from build123d import *

# Parameters (mm, degrees)
F1_DEPTH = 7.5
F3_D     = 6.6
F3_DEPTH = 4
F3_TIP   = 1.9828400428


# Not quite as in the source:
# - a pattern or mirror of a feature is missing from the dataset's text; its kind, count and spacing are read off the source's solid


with BuildPart() as f1:
    # F0 (on Right) → F1 (new body, symmetric)
    with BuildSketch(Plane.YZ):
        with BuildLine():
            Line((19.0101097905, 11), (-19.0101097905, 11))
            ThreePointArc((-19.0101097905, 11), (-30.0101097905, 0), (-19.0101097905, -11))
            Line((-19.0101097905, -11), (19.0101097905, -11))
            ThreePointArc((19.0101097905, -11), (30.0101097905, 0), (19.0101097905, 11))
        make_face()
        with BuildLine():
            Line((16.508441914, -7.5), (-16.508441914, -7.5))
            ThreePointArc((-16.508441914, -7.5), (0, -2.3140263028), (16.508441914, -7.5))
        make_face(mode=Mode.SUBTRACT)
        with BuildLine():
            ThreePointArc((-19.0101097905, -7.5), (-26.5101097905, 0), (-19.0101097905, 7.5))
            ThreePointArc((-19.0101097905, 7.5), (0, 0.8140263028), (19.0101097905, 7.5))
            ThreePointArc((19.0101097905, 7.5), (26.5101097905, 0), (19.0101097905, -7.5))
            ThreePointArc((19.0101097905, -7.5), (0, -0.8140263028), (-19.0101097905, -7.5))
        make_face(mode=Mode.SUBTRACT)
        with BuildLine():
            ThreePointArc((16.508441914, 7.5), (0, 2.3140263028), (-16.508441914, 7.5))
            Line((-16.508441914, 7.5), (16.508441914, 7.5))
        make_face(mode=Mode.SUBTRACT)
    extrude(amount=F1_DEPTH, both=True)

    # F3
    with Locations(Plane.XY.offset(11)):
        with Locations((0, 0)):
            f3 = Hole(F3_D / 2, depth=F3_DEPTH)
            with Locations((0, 0, -(F3_DEPTH + F3_TIP / 2))):  # 118° drill point
                Cone(0, F3_D / 2, F3_TIP, mode=Mode.SUBTRACT)

    # F3_copies: F3 across plane
    add(f3.mirror(Plane(origin=(0, 0, 0), x_dir=(-1, 0, 0), z_dir=(0, 0, -1))), mode=Mode.SUBTRACT)


solid = f1.part
For this review, take the finished solid that the model builds, in its own axes (mm). A direction names the side the tool comes from. Round coordinates to 2 decimals unless told otherwise and drop trailing zeros. Order: outer loops, then holes, each group sorted by start corner. A loop starts at its lowest first (then second) coordinate and runs counter-clockwise, first axis right, second up. Notation, with made-up numbers: M -27,-1.5 L -7,-1.5 A24 cw -7,35.5 Z; hole C 29.25,-20.5 d5. An arc over 180 degrees is marked long. Use a Markdown table: item, result. Add a question column.
Item 1: Mouldability with a two-part tool opening along Z and no side actions: class faces 6 (the cylindrical face through (0.105, 0.288, -0.815)), 7 (the cylindrical face through (0.105, -30.007, 0.242)), 8 (the flat face through (-7.5, 0, -2)) as released by +Z, released by -Z, zero draft, split by the parting line, or undercut.
Item 2: To check wall thickness, follow line 1 along Z through (x, y) = (4.75, -0.5); line 2 along Y through (x, z) = (-4.75, -6.75); line 3 along Y through (x, z) = (1.75, 0). State the ranges of each line that lie inside material, in increasing order.
Item 3: Add section C-C, the plane x = 0. Give the boundary of the cut face in (y, z), then the cut area to 3 significant figures.
Item 4: Add section A-A, the plane z = 0. Give the boundary of the cut face in (x, y), then the cut area to 3 significant figures.
Item 5: Insertion check: pin 1 (1 mm diameter, centred on x = 4.5, z = 8.5, fed in from +Y); pin 2 (4 mm diameter, centred on x = 5, z = -3, fed in from +Y); pin 3 (4 mm diameter, centred on x = 0, y = 0, fed in from -Z). Each pin has a flat end and moves straight along its axis. Give the tip position at first contact, or say it passes through.
Item 6: Add section B-B, the plane y = 0. Give the boundary of the cut face in (x, z).
Item 7: Tool access review of faces 1 (the cylindrical face through (2.43, 2.23, 9.23)), 2 (the flat face through (3.44, -0.27, -11)), 3 (the cylindrical face through (0.11, 26.51, 0.16)), 4 (the flat face through (7.5, 0, -2)), 5 (the cylindrical face through (2.43, 2.23, -9.23)): name each direction out of +Z, -Z, +X, -X, +Y, -Y from which nothing blocks a thin tool from reaching the whole face with its end or side.
Item 8: Add section D-D, the plane z = -6.5. Give the boundary of the cut face in (x, y), then the cut area to 3 significant figures.
Geometry results:
| question | item | result |
|---|---|---|
| 1 | face 6 | undercut |
| 1 | face 7 | split by the parting line |
| 1 | face 8 | zero draft |
| 2 | line 1 | z = -11 to -7.5, -2.32 to -0.82, 0.82 to 2.32, 7.5 to 11 |
| 2 | line 2 | y = -27.7 to -22.28, -18.04 to -15.38, 15.38 to 18.04, 22.28 to 27.7 |
| 2 | line 3 | y = -30.01 to -26.51, 26.51 to 30.01 |
| 3 | outline | M -19.01,-11 L -3.3,-11 L -3.3,-7.5 L -16.51,-7.5 A28.87 cw 16.51,-7.5 L 3.3,-7.5 L 3.3,-11 L 19.01,-11 A11 ccw 19.01,11 L 3.3,11 L 3.3,7.5 L 16.51,7.5 A28.87 cw -16.51,7.5 L -3.3,7.5 L -3.3,11 L -19.01,11 A11 ccw Z; hole M -19.01,-7.5 A30.37 cw 19.01,-7.5 A7.5 ccw 19.01,7.5 A30.37 cw -19.01,7.5 A7.5 ccw Z |
| 3 | area | 538 mm² |
| 4 | outline | M -7.5,-30.01 L 7.5,-30.01 L 7.5,-26.51 L -7.5,-26.51 Z; M -7.5,26.51 L 7.5,26.51 L 7.5,30.01 L -7.5,30.01 Z |
| 4 | area | 105 mm² |
| 5 | pin 1 | stops at y = 26.56 |
| 5 | pin 2 | stops at y = 29.96 |
| 5 | pin 3 | stops at z = -2.38 |
| 6 | outline | M -7.5,-11 L -3.3,-11 L -3.3,-7.5 L -7.5,-7.5 Z; M -7.5,-2.31 L 7.5,-2.31 L 7.5,-0.81 L -7.5,-0.81 Z; M -7.5,0.81 L 7.5,0.81 L 7.5,2.31 L -7.5,2.31 Z; M -7.5,7.5 L -3.3,7.5 L -3.3,11 L -7.5,11 Z; M 3.3,-11 L 7.5,-11 L 7.5,-7.5 L 3.3,-7.5 Z; M 3.3,7.5 L 7.5,7.5 L 7.5,11 L 3.3,11 Z |
| 7 | face 1 | +Z |
| 7 | face 2 | -Z, +X, -X, +Y, -Y |
| 7 | face 3 | +X, -X |
| 7 | face 4 | +Z, -Z, +X, +Y, -Y |
| 7 | face 5 | -Z |
| 8 | outline | M -7.5,-27.88 L 7.5,-27.88 L 7.5,-22.75 L -7.5,-22.75 Z; M -7.5,-17.69 L 7.5,-17.69 L 7.5,-14.97 L -7.5,-14.97 Z; M -7.5,14.97 L 7.5,14.97 L 7.5,17.69 L -7.5,17.69 Z; M -7.5,22.75 L 7.5,22.75 L 7.5,27.88 L -7.5,27.88 Z |
| 8 | area | 236 mm² |
